```python
from build123d import *

# Parameters (mm, degrees)
F0_R            = 19
F1_DEPTH        = 6.4
F2_R            = 1.25
F3_DEPTH        = 25.4
F3_COPIES_COUNT = 3
F4_R            = 5.25
F5_DEPTH        = 6.401


# Not quite as in the source:
# - a pattern or mirror of a feature is missing from the dataset's text; its kind, count and spacing are read off the source's solid


with BuildPart() as f1:
    # F0 (on Front) → F1 (new body)
    with BuildSketch(Plane.XZ):
        Circle(F0_R)
    extrude(amount=F1_DEPTH)

    # F2 (on Front) → F3 (cut)
    with BuildSketch(Plane.XZ):
        with Locations((5.3033008589, 5.3033008589)):
            Circle(F2_R)
    f3 = extrude(amount=F3_DEPTH, mode=Mode.SUBTRACT)

    # F3_copies: F3 ×3 about axis
    f3_copies_axis = Axis((0, 0, 0), (0, 1, 0))
    for i in range(1, F3_COPIES_COUNT):
        add(f3.rotate(f3_copies_axis, i * 360 / F3_COPIES_COUNT), mode=Mode.SUBTRACT)

    # F4 (on Front) → F5 (cut, through all)
    with BuildSketch(Plane.XZ):
        Circle(F4_R)
    extrude(amount=F5_DEPTH, mode=Mode.SUBTRACT)


solid = f1.part
```
The listing builds one solid part. Answer for the finished solid, in the listing's coordinates (mm). Give positions to 0.01 mm unless a question says otherwise; leave off trailing zeros. Write each loop counter-clockwise with the first axis right and the second up, starting at its lowest first coordinate (ties: lowest second). Pieces come first, ordered by that corner, then holes. Notation, with made-up numbers: (16.5, 82) - (60.5, 82) arc R13 cw to (60.5, 96) - close; hole circle Ø9 at (52.5, 55.25). An arc over 180 degrees is marked (long way). Use one line per item in the form item = value. Start each with the question number.
1) Find section D-D on x = 13. Determine the outline of the cut face in (y, z), plus the area to 3 significant figures.
2) The mould has two halves that part along Z. Classify faces 1 (the face through (4, -6.4, -4)), 2 (the face through (8.767, -3.155, -16.856)), 3 (the face through (-7.52, -3.16, 0.72)): pulls with the +Z half, pulls with the -Z half, needs draft (parallel to the pull), parting line crosses it, or undercut.
3) Find section A-A on z = 0. Determine the outline of the cut face in (x, y).
4) Find section C-C on y = -1.5. Determine the outline of the cut face in (x, z), plus the area to 3 significant figures.
5) Consider line 1 along X through (y, z) = (-4, 4.5); line 2 along Z through (x, y) = (1, -4); line 3 along Z through (x, y) = (-7, -3). Determine where each line is inside the solid, lowest interval first. Write a range as from..to.
6) Find section B-B on x = 0. Determine the outline of the cut face in (y, z).
Geometry results:
q1.outline = (-6.4, -13.86) - (0, -13.86) - (0, 13.86) - (-6.4, 13.86) - close
q1.area = 177 mm2
q2.face_1 = needs draft
q2.face_2 = parting line crosses it
q2.face_3 = undercut
q3.outline = (-19, -6.4) - (-5.25, -6.4) - (-5.25, 0) - (-19, 0) - close; (5.25, -6.4) - (19, -6.4) - (19, 0) - (5.25, 0) - close
q4.outline = circle Ø38 at (0, 0); hole circle Ø2.5 at (-7.24, 1.94); hole circle Ø10.5 at (0, 0); hole circle Ø2.5 at (1.94, -7.24); hole circle Ø2.5 at (5.3, 5.3)
q4.area = 1,030 mm2
q5.line_1 = -18.46..-2.7, 2.7..4.35, 6.26..18.46
q5.line_2 = -18.97..-8.07, -6.42..-5.15, 5.15..18.97
q5.line_3 = -17.66..0.72, 3.17..17.66
q6.outline = (-6.4, -19) - (0, -19) - (0, -5.25) - (-6.4, -5.25) - close; (-6.4, 5.25) - (0, 5.25) - (0, 19) - (-6.4, 19) - close
